Part model, mm, in its own coordinate system. A direction names the side the tool comes from. Round coordinates to 2 decimals unless told otherwise and drop trailing zeros. Loops run counter-clockwise (first coordinate to the right, second up) from the corner with the lowest first, then second, coordinate; pieces in that order, holes last.
(1) Tool access for faces 1 (the face through (-11.926, -0.525, 7.058)), 2 (the face through (15.75, 0.07, 3.99)), 3 (the face through (34, 11.938, 4)): list every direction of +Z, -Z, +X, -X, +Y, -Y with a clear straight run to the whole face (end or side of a thin tool).
(2) Flat gauge pins, fed straight in: pin 1 (6 mm diameter, centred on x = 140.5, z = 7.5, fed in from +Y); pin 2 (3 mm diameter, centred on x = 8.5, y = -0.5, fed in from -Z); pin 3 (1 mm diameter, centred on y = 4, z = 6.5, fed in from -X); pin 4 (2 mm diameter, centred on x = 144.5, y = 4, fed in from +Z). Where does each tip first touch, or does it go through?
(3) Probe probe 1 along X at (y, z) = (-0.25, 4.75); probe 2 along Y at (x, z) = (0, 6.75); probe 3 along Y at (x, z) = (47.5, 4). List the from-to ranges inside material, lowest first.
(4) Cut at A-A on y = 0. List the corners of the cut face in (x, z), then the cut area to 3 significant figures.
(5) Cut at C-C on z = 5. List the corners of the cut face in (x, y).
(6) Cut at D-D on x = 173. List the corners of the cut face in (y, z), then the cut area to 3 significant figures.
(7) Cut at B-B on x = 66. List the corners of the cut face in (y, z).
(8) Mould opens along Y. For faces 4 (the face through (5, -5, 11.684)), 5 (the face through (53, -3.302, 4)), 6 (the face through (177.735, 0.179, 3.992)), 7 (the face through (34, -11.938, 4)) say: +Y half, -Y half, draft (parallel to the pull), parting line (faces both ways), or undercut.
Autodesk Inventor part; units mm, degrees
ref_plane "Work Plane1" through (0, 0, 3.937) normal (0, 0, 1) x (1, 0, 0)
ref_plane "YZ Plane" through (0, 0, 0) normal (1, 0, 0) x (0, 1, 0)
ref_plane "XZ Plane" through (0, 0, 0) normal (0, 1, 0) x (-1, 0, 0)
sketch "Sketch1" plane through (0, 0, 0) normal (0, 0, 1) x (1, 0, 0)
  circle A0 centre (0, 0) radius 11.938
  line L0 (0, -11.938) -> (69.088, -11.938)
  line L1 (0, 11.938) -> (69.088, 11.938)
  line L2 (69.088, 11.938) -> (182.0608, 8.3422)
  line L3 (69.088, -11.938) -> (182.0608, -8.3422)
  arc A1 (181.2593, -8.3677) -> (181.2593, 8.3677) centre (181.7953, 0) ccw
  dimension "d0" = 23.876
extrude "Extrusion1" add sketch "Sketch1" along normal blind 11.684 contours A0
extrude "Extrusion2" add sketch "Sketch1" along normal blind 7.874 contours A0 L1 L2 A1 L3 L0
sketch "Sketch2" plane through (0, 0, 7.874) normal (0, 0, 1) x (1, 0, 0)
  line L0 (181.2593, 8.3677) -> (69.088, 11.938)
  arc A0 (181.2593, -8.3677) -> (181.2593, 8.3677) centre (181.7953, 0) ccw
  line L1 (69.088, -11.938) -> (181.2593, -8.3677)
  line L2 (69.088, 11.938) -> (0, 11.938)
  line L3 (0, -11.938) -> (69.088, -11.938)
  line L4 (69.088, -11.938) -> (181.2593, -8.3677)
  arc A1 (181.2593, -8.3677) -> (181.2593, 8.3677) centre (181.7953, 0) ccw
  line L5 (181.2593, 8.3677) -> (69.088, 11.938)
  line L6 (69.088, 11.938) -> (0, 11.938)
  arc A2 (0, -11.938) -> (0, 11.938) centre (0, 0) ccw
  circle A3 centre (181.7953, 0) radius 4.064
  line L7 (0, 0) -> (15.748, 0) construction
  line L8 (15.748, 0) -> (19.05, 0)
  arc A4 (19.05, 3.302) -> (19.05, -3.302) centre (19.05, 0) ccw
  line L9 (19.05, 3.302) -> (85.852, 3.302)
  arc A5 (85.852, -3.302) -> (85.852, 3.302) centre (85.852, 0) ccw
  line L10 (85.852, -3.302) -> (19.05, -3.302)
  dimension "d7" = 8.128
  dimension "d8" = 15.748
  dimension "d10" = 3.302
  dimension "d11" = 66.802
extrude "Extrusion3" cut sketch "Sketch2" against normal up to next contours A3 | L9 A5 L10 A4
sketch "Sketch3" plane through (0, 0, 11.684) normal (0, 0, 1) x (1, 0, 0)
  circle A0 centre (0, 0) radius 6.477
  dimension "d14" = 12.954
extrude "Extrusion4" cut sketch "Sketch3" against normal up to next
ref_plane "Work Plane1" through (0, 0, 3.937) normal (0, 0, 1) x (1, 0, 0)
properties part number "lever"
Final values:
1. face 1: +Z
1. face 2: +Z, -Z
1. face 3: +Z, -Z, +X, -X, +Y
2. pin 1: stops at y = 9.76
2. pin 2: stops at z = 0
2. pin 3: stops at x = -11.41
2. pin 4: stops at z = 7.87
3. probe 1: x = -11.94 to -6.47, 6.47 to 15.76, 89.14 to 177.74, 185.85 to 190.18
3. probe 2: y = -11.94 to -6.48, 6.48 to 11.94
3. probe 3: y = -11.94 to -3.3, 3.3 to 11.94
4. outline: (-11.94, 0) - (-6.48, 0) - (-6.48, 11.68) - (-11.94, 11.68) - close; (6.48, 0) - (15.75, 0) - (15.75, 7.87) - (11.94, 7.87) - (11.94, 11.68) - (6.48, 11.68) - close; (89.15, 0) - (177.73, 0) - (177.73, 7.87) - (89.15, 7.87) - close; (185.86, 0) - (190.18, 0) - (190.18, 7.87) - (185.86, 7.87) - close
4. area: 889 mm2
5. outline: (0, -11.94) - (69.09, -11.94) - (181.26, -8.37) arc R8.38 ccw (long way) to (181.26, 8.37) - (69.09, 11.94) - (0, 11.94) arc R11.94 ccw to start; hole circle Ø12.95 at (0, 0); hole (19.05, -3.3) - (85.85, -3.3) arc R3.3 ccw to (85.85, 3.3) - (19.05, 3.3) arc R3.3 ccw to start; hole circle Ø8.13 at (181.8, 0)
6. outline: (-8.63, 0) - (8.63, 0) - (8.63, 7.87) - (-8.63, 7.87) - close
6. area: 136 mm2
7. outline: (-11.94, 0) - (-3.3, 0) - (-3.3, 7.87) - (-11.94, 7.87) - close; (3.3, 0) - (11.94, 0) - (11.94, 7.87) - (3.3, 7.87) - close
8. face 4: draft
8. face 5: undercut
8. face 6: undercut
8. face 7: -Y half
